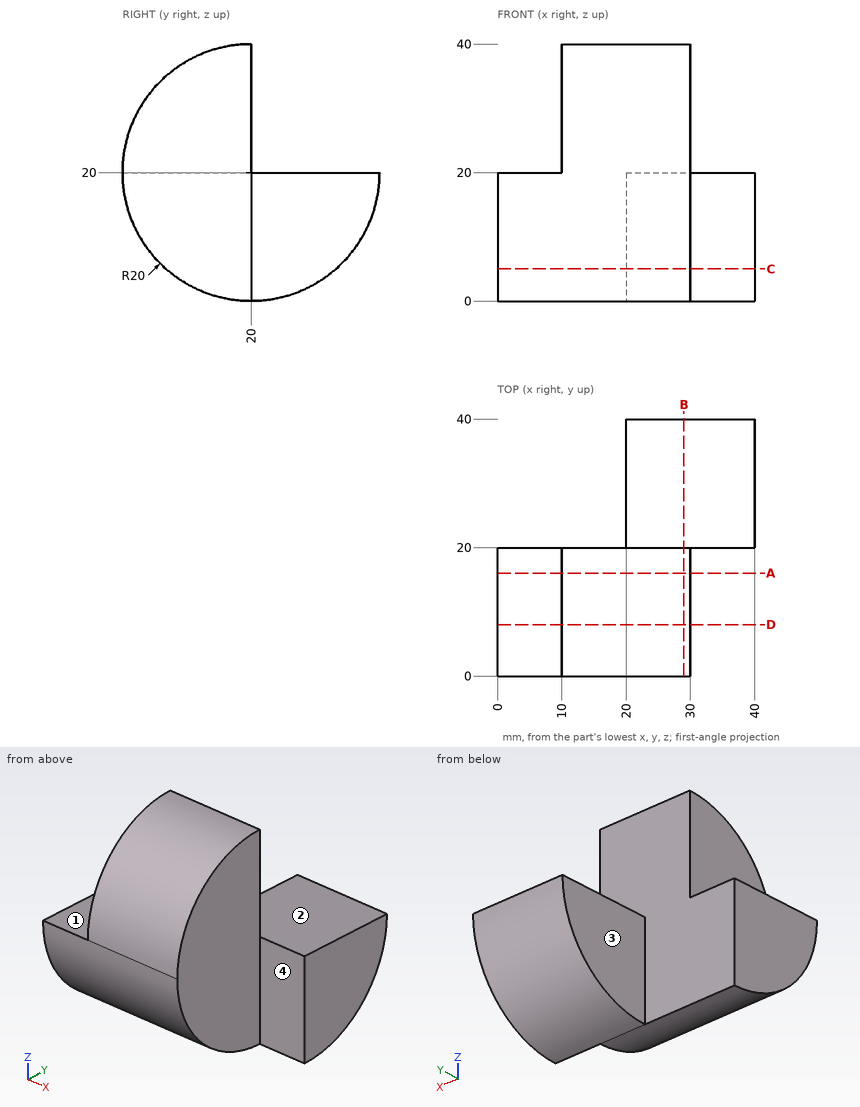
Can you work these out from the drawing? Everything is in mm from the part's minimum corner. A direction names the side the tool comes from. Coordinates: 2 decimals unless noted, no trailing zeros. Loops run counter-clockwise (first coordinate to the right, second up) from the corner with the lowest first, then second, coordinate; pieces in that order, holes last.
1) I need wall thicknesses on probe 1 along X at (y, z) = (14.5, 32); probe 2 along X at (y, z) = (25, 17.5); probe 3 along Y at (x, z) = (35, 19.5). Which ranges of each line are inside material? Lowest first, please.
2) Imagine slicing it at C-C on z = 5. List the corners of the cut face in (x, y) for me, plus the area to 3 significant figures.
3) For pin 1 (1 mm diameter, centred on x = 22, y = 12, fed in from -Z); pin 2 (3 mm diameter, centred on y = 10, z = 35.5, fed in from -X); pin 3 (6 mm diameter, centred on y = 27.5, z = 11, fed in from -X), each with a flat end and sliding along its axis, tell me the tip position at first contact or that it passes through.
4) Imagine slicing it at B-B on x = 29. List the corners of the cut face in (y, z) for me.
5) Imagine slicing it at D-D on y = 8. List the corners of the cut face in (x, z) for me.
6) Imagine slicing it at A-A on y = 16. List the corners of the cut face in (x, z) for me, plus the area to 3 significant figures.
7) Which directions (+Z, -Z, +X, -X, +Y, -Y) give clear straight access to the entire face, cutting with the end or side of a thin tool? Please do the marked faces 1, 2, 3 and 4.
Completed:
1. probe 1: x = 10 to 30
1. probe 2: x = 20 to 40
1. probe 3: y = 20 to 39.99
2. outline: (0, 6.77) - (30, 6.77) - (30, 20) - (40, 20) - (40, 33.23) - (20, 33.23) - (20, 20) - (0, 20) - close
2. area: 661 mm2
3. pin 1: stops at z = 1.46
3. pin 2: stops at x = 10
3. pin 3: stops at x = 20
4. outline: (20, 20) - (20, 40) arc R20 ccw (long way) to (40, 20) - close
5. outline: (0, 4) - (30, 4) - (30, 36) - (10, 36) - (10, 20) - (0, 20) - close
6. outline: (0, 0.4) - (30, 0.4) - (30, 39.6) - (10, 39.6) - (10, 20) - (0, 20) - close
6. area: 980 mm2
7. face 1: +Z, -X, +Y, -Y
7. face 2: +Z, +X, -X, +Y
7. face 3: +Z, -Z, -X, +Y
7. face 4: +Z, -Z, +X, -Y
